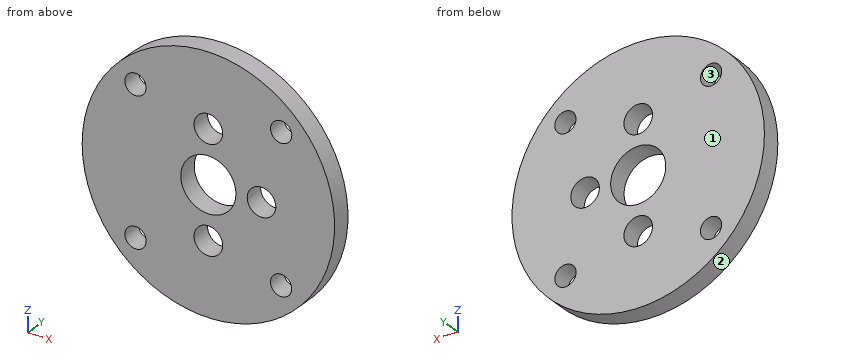
Autodesk Inventor part; units mm, degrees
ref_plane "YZ Plane" through (0, 0, 0) normal (1, 0, 0) x (0, 1, 0)
ref_plane "XZ Plane" through (0, 0, 0) normal (0, 1, 0) x (-1, 0, 0)
ref_plane "XY Plane" through (0, 0, 0) normal (0, 0, 1) x (1, 0, 0)
sketch "スケッチ1" plane through (0, 0, 0) normal (0, 1, 0) x (-1, 0, 0)
  circle A0 centre (0, 0) radius 19
  line L0 (0, 0) -> (0, 8)
  line L1 (0, 0) -> (-8, 0)
  line L2 (0, 0) -> (0, -8)
  circle A1 centre (0, -8) radius 2.15
  circle A2 centre (0, 8) radius 2.15
  circle A3 centre (-8, 0) radius 2.15
  dimension "d0" = 38
  dimension "d1" = 8
  dimension "d2" = 8
  dimension "d4" = 8
  dimension "d5" = 4.3
  dimension "d6" = 4.3
  dimension "d7" = 4.3
extrude "押し出し1" add sketch "スケッチ1" along normal blind 3
sketch "スケッチ3" plane through (0, 3, 0) normal (0, 1, 0) x (1, 0, 0)
  circle A0 centre (0, 0) radius 4.15
  dimension "d24" = 8.3
extrude "押し出し3" cut sketch "スケッチ3" against normal blind 10
sketch "スケッチ4" plane through (0, 3, 0) normal (0, 1, 0) x (1, 0, 0)
  line L0 (0, 0) -> (-10.9602, 10.9602)
  line L1 (0, 0) -> (15.5, 0) construction
  circle A0 centre (-10.9602, 10.9602) radius 1.6
  line L2 (0, 0) -> (10.9494, 10.9709)
  circle A1 centre (10.9494, 10.9709) radius 1.6
  line L3 (0, 0) -> (-10.9731, -10.9472)
  circle A2 centre (-10.9731, -10.9472) radius 1.6
  line L4 (0, 0) -> (10.9602, -10.9602)
  line L5 (0, 0) -> (15.5, 0) construction
  circle A3 centre (10.9602, -10.9602) radius 1.6
  circle A4 centre (0, 0) radius 12.5
  dimension "d27" = 15.5
  dimension "d28" = 135
  dimension "d29" = 3.2
  dimension "d30" = 15.5
  dimension "d31" = 3.2
  dimension "d32" = 15.5
  dimension "d33" = 3.2
  dimension "d34" = 15.5
  dimension "d35" = 45
  dimension "d36" = 3.2
  dimension "d37" = 25
extrude "押し出し4" cut sketch "スケッチ4" against normal blind 10 contours A0 | A1 | A2 | A3
properties part number "フランジ"
Geometry check sheet. Reference: the model listing, model coordinates, mm. Face numbers are marked on the shaded views. Round coordinates to 2 decimals unless told otherwise and drop trailing zeros. Write each loop counter-clockwise with the first axis right and the second up, starting at its lowest first coordinate (ties: lowest second). Pieces come first, ordered by that corner, then holes.
Item 1: Material ranges on line 1 along Z through (x, y) = (0, 1.4); line 2 along X through (y, z) = (2.55, -11); line 3 along Z through (x, y) = (1, 1.95), recorded low to high.
Determined:
line 1: z = -19 to -10.15, -5.85 to -4.15, 4.15 to 5.85, 10.15 to 19
line 2: x = -15.49 to -12.56, -9.36 to 9.35, 12.55 to 15.49
line 3: z = -18.97 to -9.9, -6.1 to -4.03, 4.03 to 6.1, 9.9 to 18.97
Item 2: Go/stop test with flat-tipped pins: pin 1 Ø2.5 at (x, z) = (10.95, -10.97) entering from -Y; pin 2 Ø1 at (x, y) = (0, 1) entering from +Z. Record where each tip stops, or that it passes through.
Determined:
pin 1: passes through
pin 2: stops at z = 19
Item 3: Section check D-D (z = -8). Record the boundary of the cut face in (x, y), plus the area to 3 significant figures.
Determined:
outline: (-17.23, 0) - (-2.15, 0) - (-2.15, 3) - (-17.23, 3) - close; (2.15, 0) - (17.23, 0) - (17.23, 3) - (2.15, 3) - close
area: 90.5 mm2
Item 4: Mould release check, pull along X, two halves, no side actions. Record for the marked faces 1, 2 and 3: +X half, -X half, draft (parallel to the pull), parting line (faces both ways), or undercut.
Determined:
face 1: draft
face 2: parting line
face 3: undercut
Item 5: Section check B-B (z = 0). Record the boundary of the cut face in (x, y).
Determined:
outline: (-19, 0) - (-4.15, 0) - (-4.15, 3) - (-19, 3) - close; (4.15, 0) - (5.85, 0) - (5.85, 3) - (4.15, 3) - close; (10.15, 0) - (19, 0) - (19, 3) - (10.15, 3) - close
Item 6: Section check C-C (x = 12). Record the boundary of the cut face in (y, z).
Determined:
outline: (0, -14.73) - (3, -14.73) - (3, -12.18) - (0, -12.18) - close; (0, -9.76) - (3, -9.76) - (3, 9.74) - (0, 9.74) - close; (0, 12.18) - (3, 12.18) - (3, 14.73) - (0, 14.73) - close
Item 7: Section check A-A (x = 0). Record the boundary of the cut face in (y, z), plus the area to 3 significant figures.
Determined:
outline: (0, -19) - (3, -19) - (3, -10.15) - (0, -10.15) - close; (0, -5.85) - (3, -5.85) - (3, -4.15) - (0, -4.15) - close; (0, 4.15) - (3, 4.15) - (3, 5.85) - (0, 5.85) - close; (0, 10.15) - (3, 10.15) - (3, 19) - (0, 19) - close
area: 63.3 mm2
